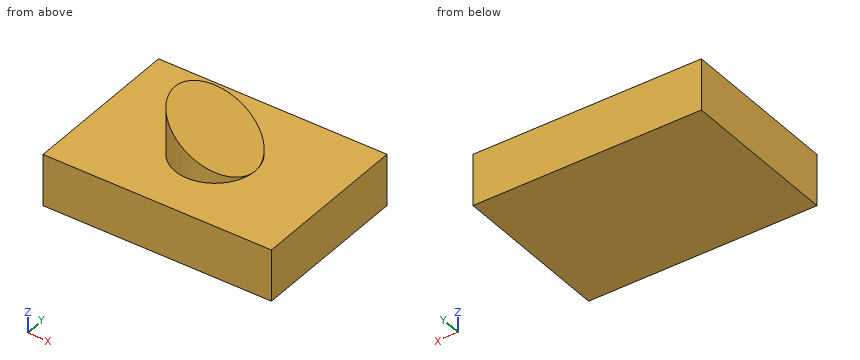
from build123d import *

# Parameters (mm, degrees)
F0_W     = 112.421236
F0_H     = 80.008708
F1_DEPTH = 25.4
F2_R     = 19.723865
F3_DEPTH = 50.8
F5_DEPTH = 80.009708


with BuildPart() as f1:
    # F0 (on Top) → F1 (new body)
    with BuildSketch(Plane.XY):
        Rectangle(F0_W, F0_H)
    extrude(amount=F1_DEPTH)

    # F2 (on Top) → F3 (join)
    with BuildSketch(Plane.XY):
        Circle(F2_R)
    extrude(amount=F3_DEPTH)

    # F4 (on face) → F5 (cut, through all)
    with BuildSketch(Plane.XZ.offset(40.004354)):
        Polygon((19.723865, 50.8), (-19.723865, 50.8), (19.723865, 25.4), align=None)
    extrude(amount=-F5_DEPTH, mode=Mode.SUBTRACT)


solid = f1.part
Model file for the job. Use its own axes, mm. Give positions to 0.01 mm unless a question says otherwise; leave off trailing zeros. Order: outer loops, then holes, each group sorted by start corner. A loop starts at its lowest first (then second) coordinate and runs counter-clockwise, first axis right, second up. Notation, with made-up numbers: (-37.5, 74) - (-30.5, 74) arc R29 cw to (-30.5, 111) - close; hole circle Ø2 at (25.25, 22). An arc over 180 degrees is marked (long way). Return JSON: item names as keys, results as strings.
1) Cut at B-B, the plane y = -31. Give the cut face in (x, z), plus the area to 3 significant figures.
Geometry says:
{"outline": "(-56.21, 0) - (56.21, 0) - (56.21, 25.4) - (-56.21, 25.4) - close", "area": "2,860 mm²"}
2) Probe line 1 (Z direction, x = 19, y = -24); line 2 (Z direction, x = -3, y = 3); line 3 (Y direction, x = 1, z = 36.5). List the from-to ranges inside material, lowest first. Write a range as from..to.
Geometry says:
{"line 1": "0..25.4", "line 2": "0..40.03", "line 3": "-19.7..19.7"}
3) Cut at A-A, the plane x = 0. Give the cut face in (y, z).
Geometry says:
{"outline": "(-40, 0) - (40, 0) - (40, 25.4) - (19.72, 25.4) - (19.72, 38.1) - (-19.72, 38.1) - (-19.72, 25.4) - (-40, 25.4) - close"}
4) Cut at C-C, the plane z = 39. Give the cut face in (x, y).
Geometry says:
{"outline": "(-1.4, -19.67) - (-1.4, 19.67) arc R19.72 ccw to start"}
5) Flat gauge pins, fed straight in: P1, Ø4, axis at x = -40, y = -21.5, coming from the -Z side; P2, Ø8, axis at x = -31.5, y = 18, coming from the +Z side; P3, Ø8, axis at x = -20.5, y = -7, coming from the +Z side. Where does each tip first touch, or does it go through?
Geometry says:
{"P1": "z = 0", "P2": "z = 25.4", "P3": "z = 50.64"}
6) Cut at D-D, the plane x = -34. Give the cut face in (y, z), plus the area to 3 significant figures.
Geometry says:
{"outline": "(-40, 0) - (40, 0) - (40, 25.4) - (-40, 25.4) - close", "area": "2,030 mm²"}
